Model file for the job. Use its own axes, mm. A direction names the side the tool comes from. Coordinates: 2 decimals unless noted, no trailing zeros. Write each loop counter-clockwise with the first axis right and the second up, starting at its lowest first coordinate (ties: lowest second). Pieces come first, ordered by that corner, then holes. Notation, with made-up numbers: (13.25, 30) -> (69.25, 30) arc R24 cw to (69.25, 52) -> close; hole circle Ø10 at (78, 40). An arc over 180 degrees is marked (long way). Answer as a JSON object with one key per item and string values. Group by question number.
from build123d import *

# Parameters (mm, degrees)
F0_W     = 200
F0_H     = 30
F1_DEPTH = 15
F2_R     = 3
F3_DEPTH = 25
F2_R_2   = 5
F4_DEPTH = 7.5


with BuildPart() as f1:
    # F0 (on Front) → F1 (new body)
    with BuildSketch(Plane.XZ):
        with Locations((54.39228, 15)):
            Rectangle(F0_W, F0_H)
    extrude(amount=F1_DEPTH)

    # F2 (on face) → F3 (cut)
    with BuildSketch(Plane.XZ.offset(15)):
        with Locations((4.39228, 15)):
            Circle(F2_R)
        with Locations((104.39228, 15)):
            Circle(F2_R)
    extrude(amount=-F3_DEPTH, mode=Mode.SUBTRACT)

    # F2 (on face) → F4 (cut)
    with BuildSketch(Plane.XZ.offset(15)):
        with Locations((4.39228, 15)):
            Circle(F2_R_2)
        with Locations((4.39228, 15)):
            Circle(F2_R, mode=Mode.SUBTRACT)
        with Locations((104.39228, 15)):
            Circle(F2_R_2)
        with Locations((104.39228, 15)):
            Circle(F2_R, mode=Mode.SUBTRACT)
    extrude(amount=-F4_DEPTH, mode=Mode.SUBTRACT)


solid = f1.part
(1) Cut at B-B on y = -10.25. List the corners of the cut face in (x, z), plus the area to 3 significant figures.
(2) 3-axis set-ups, long thin cutter, end or side, ignore diameter. For faces 1 (the face through (7, -7.5, 13)), 2 (the face through (-45.608, -7, 15)): which of +Z, -Z, +X, -X, +Y, -Y reach the whole face in a straight line?
(3) Pull direction Z, two halves, no side cores. Call faces 3 (the face through (3.74, -3.8, 12.07)), 4 (the face through (53, 0, 15)), 5 (the face through (53, -7, 30)), 6 (the face through (109.01, -11.3, 13.08)): released by +Z, released by -Z, zero draft, split by the parting line, or undercut.
(4) Wall check: probe 1 along X at (y, z) = (-13.75, 19); probe 2 along Y at (x, z) = (108, 14). Give the ranges that are in metal, low to high.
(5) Cut at C-C on x = 104. List the corners of the cut face in (y, z), plus the area to 3 significant figures.
(6) Cut at A-A on z = 15. List the corners of the cut face in (x, y), plus the area to 3 significant figures.
(7) Pin check, flat tip, straight feed: pin 1 (5 mm diameter, centred on x = 5, z = 15.5, fed in from -Y). Stop position of the tip, or through.
Results found:
{
 "1": {"outline": "(-45.61, 0) -> (154.39, 0) -> (154.39, 30) -> (-45.61, 30) -> close; hole circle Ø10 at (4.39, 15); hole circle Ø10 at (104.39, 15)", "area": "5,840 mm²"},
 "2": {"face 1": "-Y", "face 2": "+Z, -Z, -X, +Y, -Y"},
 "3": {"face 3": "undercut", "face 4": "zero draft", "face 5": "released by +Z", "face 6": "undercut"},
 "4": {"probe 1": "x = -45.61 to 1.39, 7.39 to 101.39, 107.39 to 154.39", "probe 2": "y = -7.5 to 0"},
 "5": {"outline": "(-15, 0) -> (0, 0) -> (0, 12.03) -> (-7.5, 12.03) -> (-7.5, 10.02) -> (-15, 10.02) -> close; (-15, 19.98) -> (-7.5, 19.98) -> (-7.5, 17.97) -> (0, 17.97) -> (0, 30) -> (-15, 30) -> close", "area": "331 mm²"},
 "6": {"outline": "(-45.61, -15) -> (-0.61, -15) -> (-0.61, -7.5) -> (1.39, -7.5) -> (1.39, 0) -> (-45.61, 0) -> close; (7.39, -7.5) -> (9.39, -7.5) -> (9.39, -15) -> (99.39, -15) -> (99.39, -7.5) -> (101.39, -7.5) -> (101.39, 0) -> (7.39, 0) -> close; (107.39, -7.5) -> (109.39, -7.5) -> (109.39, -15) -> (154.39, -15) -> (154.39, 0) -> (107.39, 0) -> close", "area": "2,760 mm²"},
 "7": {"pin 1": "stops at y = -7.5"}
}
